Can you work these out from the model? Positions are in its coordinate system, mm. A direction names the side the tool comes from. Give positions to 0.01 mm unless a question says otherwise; leave off trailing zeros. Write each loop counter-clockwise with the first axis right and the second up, starting at its lowest first coordinate (ties: lowest second). Pieces come first, ordered by that corner, then holes. Notation, with made-up numbers: M 4,0 L 24,0 A10 ccw 24,8 Z; hole C 88.5,-13 d7. An arc over 180 degrees is marked long. Answer as CSV lines item,"result". Start each with the question number.
Autodesk Inventor part; units mm, degrees
ref_plane "Work Plane1" through (0, 9.5179, 76.2) normal (-0.0386902, 0.9992513, 0) x (-0.9992513, -0.0386902, 0)
ref_plane "YZ Plane" through (0, 0, 0) normal (1, 0, 0) x (0, 1, 0)
ref_plane "XZ Plane" through (0, 0, 0) normal (0, 1, 0) x (-1, 0, 0)
sketch "Sketch1" plane through (0, 0, 0) normal (0, 0, 1) x (1, 0, 0)
  circle A0 centre (0.3685, 0) radius 9.525
  circle A1 centre (0.3685, 0) radius 6.985
  point P0 (0, 0)
  dimension "d0" = 19.05
  dimension "d1" = 2.54
extrude "Extrusion1" add sketch "Sketch1" along normal blind 76.2
sketch "Sketch2" plane through (0.3685, 0, 76.2) normal (0, 0, 1) x (1, 0, 0)
  circle A0 centre (0, 0) radius 6.985
  circle A1 centre (0, 0) radius 9.525
  point P0 (-0.3685, 0)
  point P1 (-0.3685, 9.5179)
ref_plane "Work Plane1" through (0, 9.5179, 76.2) normal (-0.0386902, 0.9992513, 0) x (-0.9992513, -0.0386902, 0)
sketch "Sketch3" plane through (0, 9.5179, 76.2) normal (-0.0386902, 0.9992513, 0) x (-0.9992513, -0.0386902, 0)
  line L0 (0.3682, 0.0009) -> (0.3682, -76.2) construction
  circle A0 centre (0.3682, -38.0996) radius 8.255
  dimension "d4" = 16.51
extrude "Extrusion2" add sketch "Sketch3" along normal blind 101.6 and the other way blind 6.35
sketch "Sketch4" plane through (0.3685, 0, 76.2) normal (0, 0, 1) x (1, 0, 0)
  line L0 (-1.5078, -6.8203) -> (-1.5078, -9.4049)
  line L1 (1.4136, -9.4195) -> (1.4136, -6.8405)
  arc A0 (-1.5078, -9.4049) -> (1.4136, -9.4195) centre (0, 0) ccw
  arc A1 (1.4136, -6.8405) -> (-1.5078, -6.8203) centre (0, 0) ccw
extrude "Extrusion3" cut sketch "Sketch4" against normal blind 101.6
properties part number "centerSpike" material "Iron, Cast"
1) I want a section at A-A, the plane y = 0. Please give me the cut outline in (x, z), then the cut area to 3 significant figures.
2) Thinking about a two-plate mould opening in X: for faces 5 (the flat face through (-1.139, -8, 39)), 6 (the flat face through (-4.183, 111.032, 38.216)), 7 (the flat face through (1.03, 7.11, 76.2)), which applies, released by +X, released by -X, zero draft, split by the parting line, or undercut?
3) I'm going to push flat-ended pins straight in: P1, Ø10, axis at y = 75, z = 48, coming from the -X side; P2, Ø2, axis at y = -8, z = 30, coming from the +X side; P3, Ø2, axis at x = -3, y = 31.5, coming from the +Z side. Where does each tip first touch, or does it pass through?
4) On a 3-axis mill with a long thin cutter (end or side, diameter ignored), from which of +Z, -Z, +X, -X, +Y, -Y can I reach the whole of each face in a straight line? I mean faces 1 (the cylindrical face through (0.206, 6.983, 38.216)), 2 (the flat face through (1.03, 7.11, 0)), 3 (the cylindrical face through (9.523, 2.63, 37.567)), 4 (the flat face through (1.782, -8, 39)). Say none if no direction works.
5) I need wall thicknesses on L1, parallel to X at y = 0, z = 20; L2, parallel to X at y = -0.5, z = 20; L3, parallel to Y at x = 3.25, z = 51.5. Which ranges of each line are inside material? Lowest first, please. Write a range as from..to.
Values found:
1,outline,"M -9.16,0 L -6.62,0 L -6.62,76.2 L -9.16,76.2 Z; M 7.35,0 L 9.89,0 L 9.89,76.2 L 7.35,76.2 Z"
1,area,"387 mm²"
2,face 5,"undercut"
2,face 6,"released by -X"
2,face 7,"zero draft"
3,P1,"stops at x = -9.56"
3,P2,"stops at x = 6.83"
3,P3,"stops at z = 46.32"
4,face 1,"+Z, -Z"
4,face 2,"-Z, +X, -X, +Y, -Y"
4,face 3,"none"
4,face 4,"+Z, -Z, -Y"
5,L1,"x = -9.16..-6.62, 7.35..9.89"
5,L2,"x = -9.14..-6.6, 7.34..9.88"
5,L3,"y = -9.08..-6.36, 6.36..9.08"
